Input: dimensioned drawing with shaded views. Units: mm. Origin: part minimum x, y, z. A direction names the side the tool comes from. Round coordinates to 2 decimals unless told otherwise and drop trailing zeros. Order: outer loops, then holes, each group sorted by start corner. A loop starts at its lowest first (then second) coordinate and runs counter-clockwise, first axis right, second up.
Item 1: Mould query, pull axis Y, two halves, no side actions, for the marked faces 4, 5 and 6. Classes: released by +Y, released by -Y, zero draft, split by the parting line, or undercut.
Item 2: Line query: L1, parallel to Y at x = 10.15, z = 4.15; L2, parallel to X at y = 11.5, z = 3.85; L3, parallel to X at y = 18, z = 3.35. Output: solid intervals per line, ascending.
Item 3: Cut plane A-A on x = 10.15. Output: boundary loops of the cut face in (y, z), then the cut area to 3 significant figures.
Item 4: Reachability of the marked faces 1, 2 and 3 from +Z, -Z, +X, -X, +Y, -Y: full face, straight path, thin tool, end or side. Return the list, or none.
Item 5: Cut plane B-B on y = 10. Output: boundary loops of the cut face in (x, z), then the cut area to 3 significant figures.
Item 6: Cut plane D-D on y = 39. Output: boundary loops of the cut face in (x, z).
Item 7: First-contact query: pin 1 (1.5 mm diameter, centred on y = 12.5, z = 2, fed in from +X); pin 2 (2 mm diameter, centred on x = 18, z = 2.5, fed in from -Y); pin 3 (1.8 mm diameter, centred on y = 40, z = 2, fed in from +X); pin 4 (10 mm diameter, centred on x = 29.5, y = 12, fed in from -Z). Flat tips, straight axial feed; report the tip coordinate or a pass-through.
Item 8: Cut plane C-C on z = 3.35. Output: boundary loops of the cut face in (x, y), then the cut area to 3 significant figures.
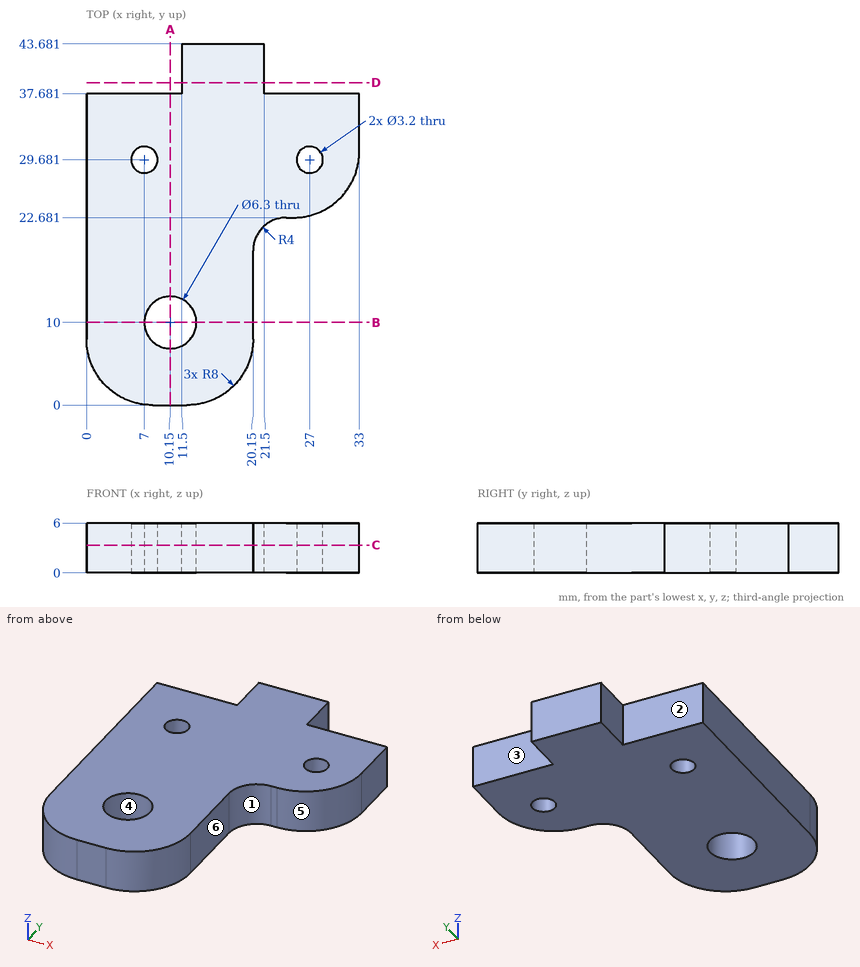
From the geometry:
1. face 4: undercut
1. face 5: released by -Y
1. face 6: zero draft
2. L1: y = 0 to 6.85, 13.15 to 37.68
2. L2: x = 0 to 7.38, 12.92 to 20.15
2. L3: x = 0 to 20.15
3. outline: (0, 0) - (6.85, 0) - (6.85, 6) - (0, 6) - close; (13.15, 0) - (37.68, 0) - (37.68, 6) - (13.15, 6) - close
3. area: 188 mm2
4. face 1: +Z, -Z, +X, -Y
4. face 2: +Z, -Z, -X, +Y
4. face 3: +Z, -Z, +X, +Y
5. outline: (0, 0) - (7, 0) - (7, 6) - (0, 6) - close; (13.3, 0) - (20.15, 0) - (20.15, 6) - (13.3, 6) - close
5. area: 83.1 mm2
6. outline: (11.5, 0) - (21.5, 0) - (21.5, 6) - (11.5, 6) - close
7. pin 1: stops at x = 20.15
7. pin 2: stops at y = 1.64
7. pin 3: stops at x = 21.5
7. pin 4: passes through
8. outline: (0, 8) arc R8 ccw to (8, 0) - (12.15, 0) arc R8 ccw to (20.15, 8) - (20.15, 18.68) arc R4 cw to (24.15, 22.68) - (25, 22.68) arc R8 ccw to (33, 30.68) - (33, 37.68) - (21.5, 37.68) - (21.5, 43.68) - (11.5, 43.68) - (11.5, 37.68) - (0, 37.68) - close; hole circle Ø3.2 at (7, 29.68); hole circle Ø6.3 at (10.15, 10); hole circle Ø3.2 at (27, 29.68)
8. area: 927 mm2
